```python
from build123d import *

# Parameters (mm, degrees)
ESQUISSE1_W        = 88
ESQUISSE1_H        = 24
BOSS_EXTRU_1_DEPTH = 9
ESQUISSE2_W        = 4
ESQUISSE2_H        = 2.5
BOSS_EXTRU_2_DEPTH = 9
CONG_1_R           = 1


with BuildPart() as part:
    # Esquisse1 → Boss.-Extru.1 (new body)
    with BuildSketch(Plane.XY):
        with Locations((0, -12)):
            Rectangle(ESQUISSE1_W, ESQUISSE1_H)
    extrude(amount=BOSS_EXTRU_1_DEPTH)

    # Esquisse2 → Boss.-Extru.2 (add)
    with BuildSketch(Plane.XY.offset(9)):
        with Locations((-38, 1.25)):
            Rectangle(ESQUISSE2_W, ESQUISSE2_H)
        with Locations((38, 1.25)):
            Rectangle(ESQUISSE2_W, ESQUISSE2_H)
    extrude(amount=-BOSS_EXTRU_2_DEPTH)

    # Congé1
    cong_1_edges = [part.edges().sort_by_distance(p)[0] for p in [
        (-40, 2.5, 4.5),
        (-40, 0, 4.5),
        (-36, 0, 4.5),
        (-36, 2.5, 4.5),
        (40, 2.5, 4.5),
        (36, 2.5, 4.5),
        (36, 0, 4.5),
        (40, 0, 4.5),
        (-44, 0, 4.5),
        (44, 0, 4.5),
        (44, -24, 4.5),
        (-44, -24, 4.5),
    ]]
    fillet(cong_1_edges, radius=CONG_1_R)


solid = part.part
```
The model under review builds one solid part; all positions refer to its coordinate system, in mm. A direction names the side the tool comes from. Round coordinates to 2 decimals unless told otherwise and drop trailing zeros. Order: outer loops, then holes, each group sorted by start corner. A loop starts at its lowest first (then second) coordinate and runs counter-clockwise, first axis right, second up. Notation, with made-up numbers: M 59.25,42 L 87.25,42 A4 cw 87.25,46 Z; hole C -23.5,65.25 d4. An arc over 180 degrees is marked long. Use a Markdown table: item, result.
1) Insertion check: pin 1 (0.6 mm diameter, centred on x = -41.5, z = 3, fed in from +Y). The pin has a flat end and moves straight along its axis. Give the tip position at first contact, or say it passes through.
Report:
| item | result |
|---|---|
| pin 1 | y = 0 |
2) Consider section B-B (x = 29.5). Write out the cut boundary in (y, z).
Report:
| item | result |
|---|---|
| outline | M -24,0 L 0,0 L 0,9 L -24,9 Z |
3) Consider section A-A (z = 2). Write out the cut boundary in (x, y), then the cut area to 3 significant figures.
Report:
| item | result |
|---|---|
| outline | M -44,-23 A1 ccw -43,-24 L 43,-24 A1 ccw 44,-23 L 44,-1 A1 ccw 43,0 L 41,0 A1 cw 40,1 L 40,1.5 A1 ccw 39,2.5 L 37,2.5 A1 ccw 36,1.5 L 36,1 A1 cw 35,0 L -35,0 A1 cw -36,1 L -36,1.5 A1 ccw -37,2.5 L -39,2.5 A1 ccw -40,1.5 L -40,1 A1 cw -41,0 L -43,0 A1 ccw -44,-1 Z |
| area | 2,130 mm^2 |
4) Wall thickness on line 1 along Y through (x, z) = (-10, 7.5); line 2 along Y through (x, z) = (36.5, 8.75): over which ranges is each line inside the solid? List them lowest first. Write a range as [from, to].
Report:
| item | result |
|---|---|
| line 1 | [-24, 0] |
| line 2 | [-24, 2.37] |
5) Tool access review of faces 1 (the face through (-1, -24, 4)), 2 (the face through (-42, 0, 4)), 3 (the face through (42, 0, 4)), 4 (the face through (0, 0, 4)): name each direction out of +Z, -Z, +X, -X, +Y, -Y from which nothing blocks a thin tool from reaching the whole face with its end or side.
Report:
| item | result |
|---|---|
| face 1 | +Z, -Z, +X, -X, -Y |
| face 2 | +Z, -Z, -X, +Y |
| face 3 | +Z, -Z, +X, +Y |
| face 4 | +Z, -Z, +Y |
